from build123d import *

# Parameters (mm, degrees)
BOSS_EXTRUDE1_DEPTH = 6
CUT_EXTRUDE1_REACH  = 68.084
SKETCH2_R           = 2.5
SKETCH3_R           = 1.5
CUT_EXTRUDE2_DEPTH  = 67.08422656
BOSS_EXTRUDE2_DEPTH = 5
BOSS_EXTRUDE3_DEPTH = 5
CUT_EXTRUDE3_REACH  = 69.728
SKETCH6_R           = 1.5
CUT_EXTRUDE4_REACH  = 69.728


with BuildPart() as part:
    # Sketch1 → Boss-Extrude1 (new body)
    with BuildSketch(Plane(origin=(0, 0, 0), x_dir=(1, 0, 0), z_dir=(0, 1, 0))):
        with BuildLine():
            Line((-50, 14.25), (50, 14.25))
            ThreePointArc((50, 14.25), (64.25, 0), (50, -14.25))
            Line((50, -14.25), (-50, -14.25))
            ThreePointArc((-50, -14.25), (-64.25, 0), (-50, 14.25))
        make_face()
    extrude(amount=BOSS_EXTRUDE1_DEPTH)

    # Sketch2 → Cut-Extrude1 (cut, up to next)
    with BuildSketch(Plane(origin=(0, 6, 0), x_dir=(1, 0, 0), z_dir=(0, 1, 0)), mode=Mode.PRIVATE) as cut_extrude1_sk1:
        with Locations(Location((-50, 8.25, 0), (0, 0, 270))):
            Circle(SKETCH2_R)
    cut_extrude1_tool1 = extrude(cut_extrude1_sk1.sketch, amount=-CUT_EXTRUDE1_REACH, mode=Mode.PRIVATE) & part.part
    # Sketch2 → Cut-Extrude1 (cut, up to next)
    with BuildSketch(Plane(origin=(0, 6, 0), x_dir=(1, 0, 0), z_dir=(0, 1, 0)), mode=Mode.PRIVATE) as cut_extrude1_sk2:
        with Locations(Location((-50, -8.25, 0), (0, 0, 270))):
            Circle(SKETCH2_R)
    cut_extrude1_tool2 = extrude(cut_extrude1_sk2.sketch, amount=-CUT_EXTRUDE1_REACH, mode=Mode.PRIVATE) & part.part
    add(cut_extrude1_tool1.solids().sort_by_distance((-50, 6, -8.25))[0], mode=Mode.SUBTRACT)
    add(cut_extrude1_tool2.solids().sort_by_distance((-50, 6, 8.25))[0], mode=Mode.SUBTRACT)

    # Sketch3 → Cut-Extrude2 (cut, through all)
    with BuildSketch(Plane.XZ):
        with Locations(Location((50, 0, 0), (0, 0, 270))):
            Circle(SKETCH3_R)
    extrude(amount=-CUT_EXTRUDE2_DEPTH, mode=Mode.SUBTRACT)

    # Sketch4 → Boss-Extrude2 (add)
    with BuildSketch(Plane(origin=(0, 6, 0), x_dir=(1, 0, 0), z_dir=(0, 1, 0))):
        with BuildLine():
            Line((-50, 14.25), (15, 14.25))
            Line((15, 14.25), (15, -14.25))
            Line((15, -14.25), (-50, -14.25))
            ThreePointArc((-50, -14.25), (-64.25, 0), (-50, 14.25))
        make_face()
    extrude(amount=BOSS_EXTRUDE2_DEPTH)

    # Sketch5 → Boss-Extrude3 (add)
    with BuildSketch(Plane(origin=(0, 11, 0), x_dir=(1, 0, 0), z_dir=(0, 1, 0))):
        with BuildLine():
            Line((-50, 14.25), (50, 14.25))
            ThreePointArc((50, 14.25), (64.25, 0), (50, -14.25))
            Line((50, -14.25), (-50, -14.25))
            ThreePointArc((-50, -14.25), (-64.25, 0), (-50, 14.25))
        make_face()
    extrude(amount=BOSS_EXTRUDE3_DEPTH)

    # Sketch6 → Cut-Extrude3 (cut, up to next)
    with BuildSketch(Plane(origin=(0, 16, 0), x_dir=(1, 0, 0), z_dir=(0, 1, 0)), mode=Mode.PRIVATE) as cut_extrude3_sk1:
        with Locations(Location((50, 0, 0), (0, 0, 90))):
            Circle(SKETCH6_R)
    cut_extrude3_tool1 = extrude(cut_extrude3_sk1.sketch, amount=-CUT_EXTRUDE3_REACH, mode=Mode.PRIVATE) & part.part
    add(cut_extrude3_tool1.solids().sort_by_distance((50, 16, 0))[0], mode=Mode.SUBTRACT)

    # Sketch7 → Cut-Extrude4 (cut, up to next)
    with BuildSketch(Plane(origin=(0, 16, 0), x_dir=(1, 0, 0), z_dir=(0, 1, 0)), mode=Mode.PRIVATE) as cut_extrude4_sk1:
        with BuildLine():
            ThreePointArc((-39.07315683, -9.146944754), (-43.970135273, -12.911360555), (-50, -14.25))
            Line((-50, -14.25), (50, -14.25))
            add(Edge.make_bspline(
                [(-39.07315683, -9.146944754), (-31.514094033, -0.116968526), (5.438655837, -4.645240543), (38.697514387, -14.25), (50, -14.25)],
                knots=[0, 0, 0, 0, 0.435907903, 1, 1, 1, 1], degree=3))
        make_face()
    cut_extrude4_tool1 = extrude(cut_extrude4_sk1.sketch, amount=-CUT_EXTRUDE4_REACH, mode=Mode.PRIVATE) & part.part
    add(cut_extrude4_tool1.solids().sort_by_distance((-8.590717, 16, 9.791359))[0], mode=Mode.SUBTRACT)


solid = part.part
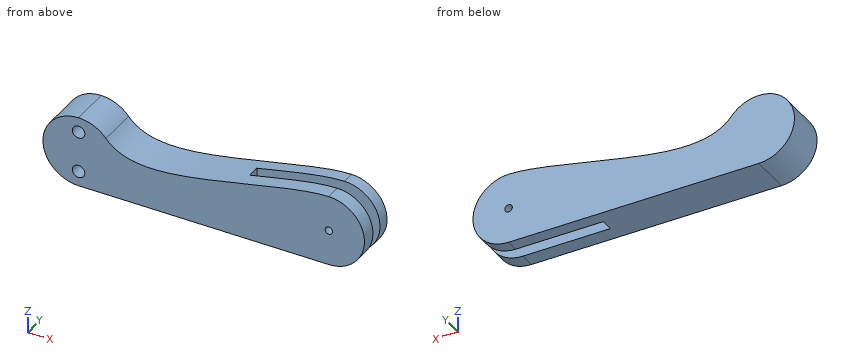
Verification items for the finished model (mm, model axes). Round coordinates to 2 decimals unless told otherwise and drop trailing zeros. Order: outer loops, then holes, each group sorted by start corner. A loop starts at its lowest first (then second) coordinate and runs counter-clockwise, first axis right, second up.
1. Go/stop test with flat-tipped pins: P1, Ø6, axis at x = 13.5, y = 11, coming from the +Z side; P2, Ø1, axis at y = 11, z = 6.5, coming from the -X side; P3, Ø4, axis at x = -50, z = 8.25, coming from the -Y side. Record where each tip stops, or that it passes through.
Final values:
P1: stops at z = 8.49
P2: stops at x = -62.93
P3: stops at y = 6
2. Section check A-A on z = 0. Record the cut outline in (x, y), then the cut area to 3 significant figures.
Final values:
outline: (-64.25, 0) - (48.5, 0) - (48.5, 6) - (15, 6) - (15, 11) - (48.5, 11) - (48.5, 16) - (-64.25, 16) - close; (51.5, 0) - (64.25, 0) - (64.25, 6) - (51.5, 6) - close; (51.5, 11) - (64.25, 11) - (64.25, 16) - (51.5, 16) - close
area: 1,780 mm2
3. Thickness scan on L1, parallel to Y at x = 39, z = 3.25; L2, parallel to X at y = 14.3, z = 0; L3, parallel to Y at x = -49, z = 9. Record the ranges inside material, lowest first.
Final values:
L1: y = 0 to 6, 11 to 16
L2: x = -64.25 to 48.5, 51.5 to 64.25
L3: y = 6 to 16
4. Section check B-B on x = 56. Record the cut outline in (y, z).
Final values:
outline: (0, -12.93) - (6, -12.93) - (6, 12.93) - (0, 12.93) - close; (11, -12.93) - (16, -12.93) - (16, 12.93) - (11, 12.93) - close
5. Section check D-D on z = -8.25. Record the cut outline in (x, y), then the cut area to 3 significant figures.
Final values:
outline: (-61.62, 0) - (-52.5, 0) - (-52.5, 6) - (-47.5, 6) - (-47.5, 0) - (61.62, 0) - (61.62, 6) - (15, 6) - (15, 11) - (61.62, 11) - (61.62, 16) - (-61.62, 16) - close
area: 1,710 mm2
6. Section check C-C on y = 3. State how many separate pieces and enclosed holes the cut face has, then the cut area to 3 significant figures.
Final values:
separate pieces: 1
enclosed holes: 3
area: 2,820 mm2
